Part model, mm, in its own coordinate system. A direction names the side the tool comes from. Give positions to 0.01 mm unless a question says otherwise; leave off trailing zeros. Write each loop counter-clockwise with the first axis right and the second up, starting at its lowest first coordinate (ties: lowest second). Pieces come first, ordered by that corner, then holes. Notation, with made-up numbers: (16, 13.25) - (36, 13.25) arc R11 cw to (36, 31.25) - close; hole circle Ø9 at (-36, 46.25). An arc over 180 degrees is marked (long way). Answer in a Markdown table with one row per item. Add a question column.
1. Pull direction Y, two halves, no side cores. Call faces 1 (the flat face through (0, -5, 11)), 2 (the cylindrical face through (-1.05, -9.47, 11.03)), 3 (the cylindrical face through (-4.5, 2.4, 10.9)), 4 (the cylindrical face through (-4.5, -12.2, 10.9)): released by +Y, released by -Y, zero draft, split by the parting line, or undercut.
2. Band-saw the part on B-B on x = -4.75. Write the cut outline in (y, z), plus the area to 3 significant figures.
3. Drop flat-ended pins along their axis: pin 1 Ø2 at (y, z) = (-6, 9.5) entering from -X; pin 2 Ø0.7 at (x, z) = (-7, 10.5) entering from +Y; pin 3 Ø2 at (x, y) = (-5, -3.5) entering from +Z. Give the stop position or say it passes through.
4. Band-saw the part on A-A on z = 15. Write the cut outline in (x, y).
5. Band-saw the part on D-D on y = -9.5. Write the cut outline in (x, z).
6. Which spindle directions (+Z, -Z, +X, -X, +Y, -Y) get a long thin tool onto all of the face, cutting with end or side? Do faces 5 (the cylindrical face through (-1.03, -0.35, 11.03)), 6 (the cylindrical face through (-4.22, -11.58, 11.17)), 7 (the flat face through (-4, -5, 5.6)). Say none if no direction does.
7. Probe line 1 along Y through (x, z) = (-4.5, 7.5); line 2 along X through (y, z) = (-7, 11.5); line 3 along Y through (x, z) = (-1.25, 13.5). List the from-to ranges inside material, lowest first.
8. Band-saw the part on C-C on y = -4. Write the cut outline in (x, z), plus the area to 3 significant figures.
```python
from build123d import *

# Parameters (mm, degrees)
F1_DEPTH = 10
F2_R     = 1.5
F4_DEPTH = 0.5
F5_ANGLE = -90


with BuildPart() as f1:
    # F0 (on Front) → F1 (new body)
    with BuildSketch(Plane.XZ):
        with BuildLine():
            Line((-2, -5.6), (0, -5.6))
            Line((0, -5.6), (0, 5.6))
            Line((0, 5.6), (-2, 5.6))
            ThreePointArc((-2, 5.6), (-4.5, 7.3), (-7, 5.6))
            Line((-7, 5.6), (-6.339597, 5.6))
            ThreePointArc((-6.339597, 5.6), (-4.181785, 6.675612), (-2.448172, 5))
            Line((-2.448172, 5), (-0.6, 5))
            Line((-0.6, 5), (-0.6, -5))
            Line((-0.6, -5), (-2.448172, -5))
            ThreePointArc((-2.448172, -5), (-4.181785, -6.675612), (-6.339597, -5.6))
            Line((-6.339597, -5.6), (-7, -5.6))
            ThreePointArc((-7, -5.6), (-4.5, -7.3), (-2, -5.6))
        make_face()
    extrude(amount=F1_DEPTH)

    # F2
    f2_edges = [f1.edges().sort_by_distance(p)[0] for p in [
        (0, -5, 5.6),
        (0, -5, -5.6),
        (-0.6, -5, 5),
        (-0.6, -5, -5),
    ]]
    fillet(f2_edges, radius=F2_R)

    # F3 (on face) → F4 (join)
    with BuildSketch(Plane.XZ.offset(10)):
        with BuildLine():
            Line((-6.339597, 5.6), (-7, 5.6))
            Line((-7, 5.6), (-7, -5.6))
            Line((-7, -5.6), (-6.339597, -5.6))
            ThreePointArc((-6.339597, -5.6), (-4.181785, -6.675612), (-2.448172, -5))
            Line((-2.448172, -5), (-2.1, -5))
            ThreePointArc((-2.1, -5), (-1.03934, -4.56066), (-0.6, -3.5))
            Line((-0.6, -3.5), (-0.6, 3.5))
            ThreePointArc((-0.6, 3.5), (-1.03934, 4.56066), (-2.1, 5))
            Line((-2.1, 5), (-2.448172, 5))
            ThreePointArc((-2.448172, 5), (-4.181785, 6.675612), (-6.339597, 5.6))
        make_face()
        with BuildLine():
            Line((-1.5, 5.6), (-2, 5.6))
            ThreePointArc((-2, 5.6), (-4.5, 7.3), (-7, 5.6))
            Line((-7, 5.6), (-6.339597, 5.6))
            ThreePointArc((-6.339597, 5.6), (-4.181785, 6.675612), (-2.448172, 5))
            Line((-2.448172, 5), (-2.1, 5))
            ThreePointArc((-2.1, 5), (-1.03934, 4.56066), (-0.6, 3.5))
            Line((-0.6, 3.5), (-0.6, -3.5))
            ThreePointArc((-0.6, -3.5), (-1.03934, -4.56066), (-2.1, -5))
            Line((-2.1, -5), (-2.448172, -5))
            ThreePointArc((-2.448172, -5), (-4.181785, -6.675612), (-6.339597, -5.6))
            Line((-6.339597, -5.6), (-7, -5.6))
            ThreePointArc((-7, -5.6), (-4.5, -7.3), (-2, -5.6))
            Line((-2, -5.6), (-1.5, -5.6))
            ThreePointArc((-1.5, -5.6), (-0.43934, -5.16066), (0, -4.1))
            Line((0, -4.1), (0, 4.1))
            ThreePointArc((0, 4.1), (-0.43934, 5.16066), (-1.5, 5.6))
        make_face()
    extrude(amount=F4_DEPTH)


with BuildPart() as f1_1:
    # F5: moved
    add(f1.part.rotate(Axis((-1.75, -10.5, 5.6), (-1, 0, 0)), F5_ANGLE))


solid = f1_1.part
```
Values:
| question | item | result |
|---|---|---|
| 1 | face 1 | zero draft |
| 1 | face 2 | undercut |
| 1 | face 3 | released by +Y |
| 1 | face 4 | released by -Y |
| 2 | outline | (-12.19, 5.6) - (2.39, 5.6) - (2.39, 16.1) - (1.78, 16.1) - (1.78, 6.1) - (-11.58, 6.1) - (-11.58, 16.1) - (-12.19, 16.1) - close |
| 2 | area | 19.4 mm² |
| 3 | pin 1 | stops at x = -0.6 |
| 3 | pin 2 | stops at y = 1.33 |
| 3 | pin 3 | stops at z = 6.1 |
| 4 | outline | (-7, -10.5) arc R2.69 ccw to (-2, -10.5) - (-1.5, -10.5) arc R1.5 ccw to (0, -9) - (0, -0.8) arc R1.5 ccw to (-1.5, 0.7) - (-2, 0.7) arc R2.69 ccw to (-7, 0.7) - (-6.34, 0.7) arc R2.09 cw to (-2.45, 0.1) - (-2.1, 0.1) arc R1.5 cw to (-0.6, -1.4) - (-0.6, -8.4) arc R1.5 cw to (-2.1, -9.9) - (-2.45, -9.9) arc R2.09 cw to (-6.34, -10.5) - close |
| 5 | outline | (-7, 5.6) - (-0.09, 5.6) - (-0.09, 16.1) - (-1.08, 16.1) - (-1.08, 6.1) - (-7, 6.1) - close |
| 6 | face 5 | +Z, -X |
| 6 | face 6 | +Z |
| 6 | face 7 | -Z, +X, -X, +Y, -Y |
| 7 | line 1 | y = -12.2 to -11.6, 1.8 to 2.4 |
| 7 | line 2 | x = -0.6 to 0 |
| 7 | line 3 | y = -10.48 to -9.64, -0.16 to 0.68 |
| 8 | outline | (-7, 5.6) - (0, 5.6) - (0, 16.1) - (-0.6, 16.1) - (-0.6, 6.1) - (-7, 6.1) - close |
| 8 | area | 9.50 mm² |
